from build123d import *

# Parameters (mm, degrees)
BOSS_EXTRU_1_START = -5.8
BOSS_EXTRU_1_DEPTH = 1.2
ESQUISSE4_R        = 7
BOSS_EXTRU_2_DEPTH = 0.5


with BuildPart() as part:
    # Esquisse2 → Révolution1 (revolve)
    with BuildSketch(Plane.XY, mode=Mode.PRIVATE) as r_volution1_sk:
        Polygon((0, 17.7), (-8.85, 17.7), (-8.85, 5), (-9.95, 5), (-9.95, 0), (-3, 0), (-3, -4), (-5, -5), (-5, -10.8), (-11.1, -10.8), (-11.1, -18.5), (0, -18.5), align=None)
    revolve(r_volution1_sk.sketch.rotate(Axis((0, -55, 0), (0, 1, 0)), 270), axis=Axis((0, -55, 0), (0, 1, 0)))

    # Esquisse3 → Boss.-Extru.1 (add)
    with BuildSketch(Plane.XZ.offset(18.5).offset(BOSS_EXTRU_1_START)):
        with BuildLine():
            Line((-9, 6.496922348), (-9, 11.9))
            Line((-9, 11.9), (9, 11.9))
            Line((9, 11.9), (9, 6.496922348))
            ThreePointArc((9, 6.496922348), (0, 11.1), (-9, 6.496922348))
        make_face()
    extrude(amount=-BOSS_EXTRU_1_DEPTH)

    # Esquisse4 → Boss.-Extru.2 (add)
    with BuildSketch(Plane(origin=(0, 17.7, 0), x_dir=(1, 0, 0), z_dir=(0, 1, 0))):
        with Locations(Location((0, 0, 0), (0, 0, 270))):
            Circle(ESQUISSE4_R)
    extrude(amount=BOSS_EXTRU_2_DEPTH)


solid = part.part
Input: part model. Units: mm. Frame: model coordinates. A direction names the side the tool comes from. Round coordinates to 2 decimals unless told otherwise and drop trailing zeros. Loops run counter-clockwise (first coordinate to the right, second up) from the corner with the lowest first, then second, coordinate; pieces in that order, holes last. Notation, with made-up numbers: M 34,39.25 L 70,39.25 A19 cw 70,69.25 Z; hole C 59,-23.5 d6. An arc over 180 degrees is marked long. Answer as CSV lines item,"result". Start each with the question number.
(1) Section A-A, the plane z = 0. Output: boundary loops of the cut face in (x, y), plus the area to 3 significant figures.
(2) Reachability of faces 5 (the flat face through (0.1, -12.7, 11.6)), 6 (the flat face through (0.1, -11.5, 11.6)), 7 (the flat face through (-3, 17.7, 7)) from +Z, -Z, +X, -X, +Y, -Y: full face, straight path, thin tool, end or side. Return the list, or none.
(3) Section C-C, the plane x = -5.5. Output: boundary loops of the cut face in (y, z).
(4) Section D-D, the plane x = 0. Output: boundary loops of the cut face in (y, z), plus the area to 3 significant figures.
(5) Line query: line 1 (Y direction, x = 0.25, z = -5.25); line 2 (Y direction, x = -8.5, z = -4.5); line 3 (X direction, y = -12.5, z = 7.25). Output: solid intervals per line, ascending. Write a range as [from, to].
(6) First-contact query: pin 1 (8 mm diameter, centred on x = -1, y = 10, fed in from -Z); pin 2 (10 mm diameter, centred on y = -4.5, z = -1.5, fed in from +X); pin 3 (1 mm diameter, centred on y = -12, z = 8.5, fed in from +X). Flat tips, straight axial feed; report the tip coordinate or a pass-through.
(7) Draft query along Y for faces 1 (the flat face through (-9, -12, 9)), 2 (the cylindrical face through (-0.9, -2.03, -2.86)), 3 (the cylindrical face through (4.88, -7.94, 1.08)), 4 (the flat face through (0, 18.2, 0)). Return one class per face: released by +Y, released by -Y, zero draft, split by the parting line, or undercut.
(8) Section B-B, the plane z = 9.5. Output: boundary loops of the cut face in (x, y).
Values found:
1,outline,"M -11.1,-18.5 L 11.1,-18.5 L 11.1,-10.8 L 5,-10.8 L 5,-5 L 3,-4 L 3,0 L 9.95,0 L 9.95,5 L 8.85,5 L 8.85,17.7 L 7,17.7 L 7,18.2 L -7,18.2 L -7,17.7 L -8.85,17.7 L -8.85,5 L -9.95,5 L -9.95,0 L -3,0 L -3,-4 L -5,-5 L -5,-10.8 L -11.1,-10.8 Z"
1,area,"592 mm²"
2,face 5,"+Z, -Y"
2,face 6,"+Z, +Y"
2,face 7,"+Y"
3,outline,"M -18.5,-9.64 L -10.8,-9.64 L -10.8,9.64 L -11.5,9.64 L -11.5,11.9 L -12.7,11.9 L -12.7,9.64 L -18.5,9.64 Z; M 0,-8.29 L 5,-8.29 L 5,-6.93 L 17.7,-6.93 L 17.7,-4.33 L 18.2,-4.33 L 18.2,4.33 L 17.7,4.33 L 17.7,6.93 L 5,6.93 L 5,8.29 L 0,8.29 Z"
4,outline,"M -18.5,-11.1 L -10.8,-11.1 L -10.8,-5 L -5,-5 L -4,-3 L 0,-3 L 0,-9.95 L 5,-9.95 L 5,-8.85 L 17.7,-8.85 L 17.7,-7 L 18.2,-7 L 18.2,7 L 17.7,7 L 17.7,8.85 L 5,8.85 L 5,9.95 L 0,9.95 L 0,3 L -4,3 L -5,5 L -10.8,5 L -10.8,11.1 L -11.5,11.1 L -11.5,11.9 L -12.7,11.9 L -12.7,11.1 L -18.5,11.1 Z"
4,area,"593 mm²"
5,line 1,"y = [-18.5, -10.8], [0, 18.2]"
5,line 2,"y = [-18.5, -10.8], [0, 5]"
5,line 3,"x = [-9, 9]"
6,pin 1,"stops at z = -8.85"
6,pin 2,"stops at x = 9.95"
6,pin 3,"stops at x = 9"
7,face 1,"zero draft"
7,face 2,"undercut"
7,face 3,"undercut"
7,face 4,"released by +Y"
8,outline,"M -9,-12.7 L -5.74,-12.7 L -5.74,-18.5 L 5.74,-18.5 L 5.74,-12.7 L 9,-12.7 L 9,-11.5 L 5.74,-11.5 L 5.74,-10.8 L -5.74,-10.8 L -5.74,-11.5 L -9,-11.5 Z; M -2.96,0 L 2.96,0 L 2.96,5 L -2.96,5 Z"
